Part model, mm, in its own coordinate system. A direction names the side the tool comes from. Give positions to 0.01 mm unless a question says otherwise; leave off trailing zeros. Write each loop counter-clockwise with the first axis right and the second up, starting at its lowest first coordinate (ties: lowest second). Pieces come first, ordered by that corner, then holes. Notation, with made-up numbers: (27, 52.25) - (42, 52.25) arc R22 cw to (42, 79.25) - close; hole circle Ø8 at (11, -2.75). An arc over 180 degrees is marked (long way). Answer in a Markdown table with one row per item. Add a question column.
1. Band-saw the part on A-A on z = -10.5. Write the cut outline in (x, y).
2. Band-saw the part on D-D on x = -31. Write the cut outline in (y, z), plus the area to 3 significant figures.
3. Probe line 1 along Z through (x, y) = (19, 18.75); line 2 along X through (y, z) = (1.9, 16); line 3 along X through (y, z) = (7.75, 20). List the from-to ranges inside material, lowest first.
4. Band-saw the part on B-B on y = 15. Write the cut outline in (x, z).
5. Band-saw the part on C-C on y = 7. Write the cut outline in (x, z).
6. Drop flat-ended pins along their axis: pin 1 Ø3 at (x, y) = (21.5, 16) entering from +Z; pin 2 Ø8 at (y, z) = (16.5, -15) entering from -X; pin 3 Ø5.5 at (y, z) = (15, -10.5) entering from -X; pin 4 Ø18.5 at (x, z) = (-25, 17) entering from +Y. Give the stop position or say it passes through.
7. Pull direction Y, two halves, no side cores. Call faces 1 (the flat face through (22, 10, -11)), 2 (the flat face through (16, 18.3, -10.3)), 3 (the cylindrical face through (14.03, 12.07, -9.85)), 4 (the flat face through (-1, 0, 0)): released by +Y, released by -Y, zero draft, split by the parting line, or undercut.
8. Which spindle directions (+Z, -Z, +X, -X, +Y, -Y) get a long thin tool onto all of the face, cutting with end or side? Do faces 5 (the flat face through (12, 18.3, -10.8)), 6 (the flat face through (-22, 8, 24.5)), 7 (the flat face through (34, 5, -6)), 8 (the flat face through (26, 15, 9)). Say none if no direction does.
```python
from build123d import *

# Parameters (mm, degrees)
SKETCH_1_W          = 80
SKETCH_1_H          = 60
EXTRUDE_1_DEPTH     = 10
SKETCH_2_R          = 5.5
SKETCH_2_R_2        = 4.5
CUT_EXTRUDE_1_DEPTH = 51.990195136
EXTRUDE_2_DEPTH     = 10
SKETCH_5_R          = 3
CUT_EXTRUDE_3_DEPTH = 67.603303221
SKETCH_6_W          = 25
SKETCH_6_H          = 17
CUT_EXTRUDE_4_DEPTH = 5


with BuildPart() as part:
    # Эскиз1 → Бобышка-Вытянуть1 (new body)
    with BuildSketch(Plane(origin=(0, 0, 0), x_dir=(1, 0, 0), z_dir=(0, 1, 0))):
        Rectangle(SKETCH_1_W, SKETCH_1_H)
    extrude(amount=EXTRUDE_1_DEPTH)

    # Эскиз2 → Вырез-Вытянуть1 (cut, through all)
    with BuildSketch(Plane(origin=(0, 10, 0), x_dir=(1, 0, 0), z_dir=(0, 1, 0))):
        with Locations(Location((-22, -16, 0), (0, 0, 270))):
            Circle(SKETCH_2_R)
        with Locations((28, 10.5)):
            Circle(SKETCH_2_R_2)
        with BuildLine():
            ThreePointArc((32.5, 10.5), (31.181980515, 7.318019485), (28, 6))
            Line((28, 6), (40, 6))
            Line((40, 6), (40, 15))
            Line((40, 15), (28, 15))
            ThreePointArc((28, 15), (31.181980515, 13.681980515), (32.5, 10.5))
        make_face()
    extrude(amount=-CUT_EXTRUDE_1_DEPTH, mode=Mode.SUBTRACT)

    # Эскиз4 → Бобышка-Вытянуть2 (add)
    with BuildSketch(Plane(origin=(0, 10, 0), x_dir=(1, 0, 0), z_dir=(0, 1, 0))):
        Polygon((40, -9), (40, -5), (16, -5), (16, 26), (40, 26), (40, 30), (12, 30), (12, -9), align=None)
    extrude(amount=EXTRUDE_2_DEPTH)

    # Эскиз5 → Вырез-Вытянуть3 (cut, through all)
    with BuildSketch(Plane(origin=(16, 0, 0), x_dir=(0, 0, -1), z_dir=(1, 0, 0))):
        with Locations((10.5, 15)):
            Circle(SKETCH_5_R)
    extrude(amount=-CUT_EXTRUDE_3_DEPTH, mode=Mode.SUBTRACT)

    # Эскиз6 → Вырез-Вытянуть4 (cut)
    with BuildSketch(Plane(origin=(0, 10, 0), x_dir=(1, 0, 0), z_dir=(0, 1, 0))):
        with Locations((-22, -16)):
            Rectangle(SKETCH_6_W, SKETCH_6_H)
    extrude(amount=-CUT_EXTRUDE_4_DEPTH, mode=Mode.SUBTRACT)


solid = part.part
```
Values:
| question | item | result |
|---|---|---|
| 1 | outline | (-40, 0) - (23.5, 0) - (23.5, 10) - (16, 10) - (16, 12) - (12, 12) - (12, 10) - (-40, 10) - close; (12, 18) - (16, 18) - (16, 20) - (12, 20) - close |
| 2 | outline | (0, -30) - (10, -30) - (10, 7.5) - (5, 7.5) - (5, 24.5) - (10, 24.5) - (10, 30) - (0, 30) - close |
| 2 | area | 515 mm² |
| 3 | line 1 | z = -30 to -26, 5 to 9 |
| 3 | line 2 | x = -40 to -27.5, -16.5 to 40 |
| 3 | line 3 | x = -40 to -34.5, -9.5 to 40 |
| 4 | outline | (12, -30) - (40, -30) - (40, -26) - (16, -26) - (16, -13.5) - (12, -13.5) - close; (12, -7.5) - (16, -7.5) - (16, 5) - (40, 5) - (40, 9) - (12, 9) - close |
| 5 | outline | (-40, -30) - (40, -30) - (40, -15) - (28, -15) arc R4.5 cw to (28, -6) - (40, -6) - (40, 30) - (-40, 30) - close; hole (-34.5, 7.5) - (-9.5, 7.5) - (-9.5, 24.5) - (-34.5, 24.5) - close |
| 6 | pin 1 | stops at z = 9 |
| 6 | pin 2 | stops at x = 12 |
| 6 | pin 3 | passes through |
| 6 | pin 4 | stops at y = 10 |
| 7 | face 1 | released by +Y |
| 7 | face 2 | zero draft |
| 7 | face 3 | undercut |
| 7 | face 4 | released by -Y |
| 8 | face 5 | +Z, -Z, -X, +Y |
| 8 | face 6 | +Y |
| 8 | face 7 | +X, +Y, -Y |
| 8 | face 8 | +Z, +X, -X, +Y |
